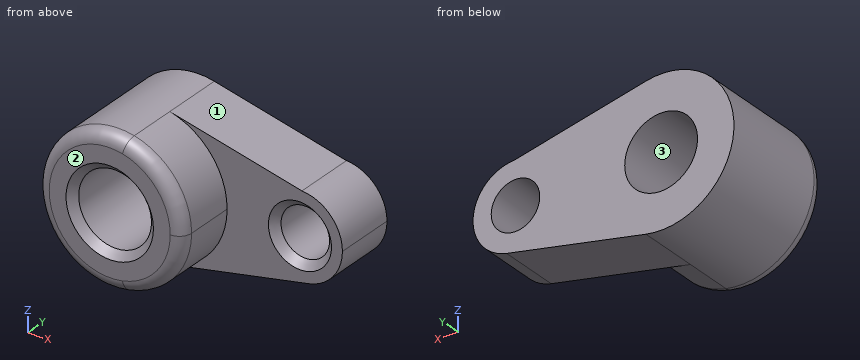
from build123d import *

# Parameters (mm, degrees)
F0_R     = 15
F0_R_2   = 10
F1_DEPTH = 25
F2_DEPTH = 50
F3_R     = 5.08
F4_SIZE  = 3


with BuildPart() as f1:
    # F0 (on Front) → F1 (new body)
    with BuildSketch(Plane.XZ):
        with BuildLine():
            ThreePointArc((6.25, -29.341736), (23.318448, -18.874586), (30, 0))
            ThreePointArc((30, 0), (23.357967, 18.825657), (6.372975, 29.315272))
            ThreePointArc((6.372975, 29.315272), (-29.999934, 0.062895), (6.25, -29.341736))
        make_face()
        Circle(F0_R, mode=Mode.SUBTRACT)
        with BuildLine():
            ThreePointArc((6.372975, 29.315272), (23.357967, 18.825657), (30, 0))
            ThreePointArc((30, 0), (23.318448, -18.874586), (6.25, -29.341736))
            Line((6.25, -29.341736), (63.645833, -17.116013))
            ThreePointArc((63.645833, -17.116013), (42.558559, -1.430429), (60.808394, 17.481319))
            Line((60.808394, 17.481319), (6.372975, 29.315272))
        make_face()
        with BuildLine():
            ThreePointArc((77.5, 0), (72.656953, 12.085179), (60.808394, 17.481319))
            ThreePointArc((60.808394, 17.481319), (42.558559, -1.430429), (63.645833, -17.116013))
            ThreePointArc((63.645833, -17.116013), (73.602428, -11.010175), (77.5, 0))
        make_face()
        with Locations((60, 0)):
            Circle(F0_R_2, mode=Mode.SUBTRACT)
    extrude(amount=F1_DEPTH)

    # F0 (on Front) → F2 (join)
    with BuildSketch(Plane.XZ):
        with BuildLine():
            ThreePointArc((6.25, -29.341736), (23.318448, -18.874586), (30, 0))
            ThreePointArc((30, 0), (23.357967, 18.825657), (6.372975, 29.315272))
            ThreePointArc((6.372975, 29.315272), (-29.999934, 0.062895), (6.25, -29.341736))
        make_face()
        Circle(F0_R, mode=Mode.SUBTRACT)
    extrude(amount=F2_DEPTH)

    # F3
    f3_edges = [f1.edges().sort_by_distance(p)[0] for p in [
        (-6.25, -50, 29.341736),
    ]]
    fillet(f3_edges, radius=F3_R)

    # F4
    f4_edges = [f1.edges().sort_by_distance(p)[0] for p in [
        (-15, -50, 0),
        (50, -25, 0),
    ]]
    chamfer(f4_edges, length=F4_SIZE)


solid = f1.part
Build history of the part. All positions in model axes, mm. Face numbers are marked on the shaded views. Coordinates: 2 decimals unless noted, no trailing zeros. Order: outer loops, then holes, each group sorted by start corner. A loop starts at its lowest first (then second) coordinate and runs counter-clockwise, first axis right, second up. Notation, with made-up numbers: (-40, -27) - (-28, -27) arc R22 ccw to (-28, -20) - close; hole circle Ø4 at (-19, -30.5). An arc over 180 degrees is marked (long way). Put each result on its own line as item: value.
1. Drop flat-ended pins along their axis: P1, Ø5, axis at y = -7, z = -0.5, coming from the -X side; P2, Ø17.5, axis at x = 41.5, z = -4.5, coming from the -Y side; P3, Ø2, axis at y = -11.5, z = -2.5, coming from the +X side. Give the stop position or say it passes through.
Answer sheet:
P1: stops at x = -30
P2: stops at y = -25
P3: stops at x = 77.44
2. Saw through at B-B (x = 33.5). Write the cut outline in (y, z).
Answer sheet:
outline: (-25, -23.54) - (0, -23.54) - (0, 23.42) - (-25, 23.42) - close
3. Pull direction X, two halves, no side cores. Call the marked faces 1, 2 and 3: pulls with the +X half, pulls with the -X half, needs draft (parallel to the pull), parting line crosses it, or undercut.
Answer sheet:
face 1: pulls with the +X half
face 2: needs draft
face 3: undercut
4. Saw through at C-C (z = -6). Give the number of separate pieces and of enclosed holes in the cut face, and give its area (3 significant figures).
Answer sheet:
separate pieces: 3
enclosed holes: 0
area: 2,310 mm^2
5. Probe line 1 along Z through (x, y) = (0, -30); line 2 along X through (y, z) = (-5, -2.5); line 3 along X through (y, z) = (-35, -3.5). List the from-to ranges inside material, lowest first. Write a range as [from, to].
Answer sheet:
line 1: z = [-30, -15], [15, 30]
line 2: x = [-29.9, -14.79], [14.79, 50.32], [69.68, 77.32]
line 3: x = [-29.8, -14.59], [14.59, 29.8]
6. Saw through at A-A (y = -33.5). Write the cut outline in (x, z), and give its area (3 significant figures).
Answer sheet:
outline: (6.25, -29.34) arc R30 ccw to (30, 0) arc R30 ccw (long way) to start; hole circle Ø30 at (0, 0)
area: 2,120 mm^2
